```python
from build123d import *

# Parameters (mm, degrees)
SKETCH1_W                      = 11
SKETCH1_H                      = 9
BOSS_EXTRUDE1_DEPTH            = 2.5
BOSS_EXTRUDE2_DEPTH            = 0.4
CUT_EXTRUDE1_DEPTH             = 12.41315031
SKETCH4_W                      = 9
SKETCH4_H                      = 11
BOSS_EXTRUDE3_DEPTH            = 2.45
SKETCH5_W                      = 9
SKETCH5_H                      = 11
BOSS_EXTRUDE4_DEPTH            = 9.45
SKETCH6_W                      = 0.9
SKETCH6_H                      = 8.5
CUT_EXTRUDE2_DEPTH             = 20.892712233
SKETCH7_W                      = 0.52
SKETCH7_H                      = 6
CUT_EXTRUDE3_DEPTH             = 18.424695119
SKETCH8_W                      = 5.62
SKETCH8_H                      = 3
BOSS_EXTRUDE5_DEPTH            = 0.36
SKETCH9_W                      = 3
SKETCH9_H                      = 2.5
BOSS_EXTRUDE6_DEPTH            = 0.52
CUT_EXTRUDE4_REACH             = 19.516
SKETCH11_W                     = 1
SKETCH11_H                     = 0.1
BOSS_EXTRUDE7_DEPTH            = 0.36
CUT_EXTRUDE5_REACH             = 20.109
SKETCH14_W                     = 0.36
SKETCH14_H                     = 1
SKETCH15_W                     = 10
SKETCH15_H                     = 4.5
CUT_EXTRUDE6_DEPTH             = 20.7068516
BOSS_EXTRUDE8_DEPTH            = 10
SKETCH17_W                     = 1.5
SKETCH17_H                     = 1.7
CUT_EXTRUDE7_DEPTH             = 20.7068516
SKETCH18_W                     = 6
SKETCH18_H                     = 1.5
BOSS_EXTRUDE9_DEPTH            = 1.5
BOSS_EXTRUDE10_DEPTH           = 0.25
F_6_5_6_5_DIAMETER_HOLE1_D     = 6.5
F_6_5_6_5_DIAMETER_HOLE1_DEPTH = 7
DRAFT1_ANGLE                   = -47
DRAFT2_ANGLE                   = 47
SKETCH22_W                     = 6
SKETCH22_H                     = 1.25
CHAMFER1_SIZE                  = 0.2


with BuildPart() as part:
    # Sketch1 → Boss-Extrude1 (new body)
    with BuildSketch(Plane(origin=(-11.95, 0, 0), x_dir=(0, -1, 0), z_dir=(-1, 0, 0))):
        with Locations((1, 0)):
            Rectangle(SKETCH1_W, SKETCH1_H)
    extrude(amount=-BOSS_EXTRUDE1_DEPTH)

    # Sketch2 → Boss-Extrude2 (add)
    with BuildSketch(Plane(origin=(0, 0, -4.5), x_dir=(-1, 0, 0), z_dir=(0, 0, -1))):
        with BuildLine():
            Line((10.2, -9.5), (10.2, -7.004276533))
            Line((10.2, -7.004276533), (9.45, -6.2))
            Line((9.45, -6.2), (9.45, 4.5))
            Line((9.45, 4.5), (11.95, 4.5))
            Line((11.95, 4.5), (11.95, -6.2))
            Line((11.95, -6.2), (11.2, -7.004276533))
            Line((11.2, -7.004276533), (11.2, -9.5))
            ThreePointArc((11.2, -9.5), (10.7, -10), (10.2, -9.5))
        make_face()
    extrude(amount=BOSS_EXTRUDE2_DEPTH)

    # Sketch3 → Cut-Extrude1 (cut, through all)
    with BuildSketch(Plane(origin=(-9.45, 0, 0), x_dir=(0, 0, -1), z_dir=(1, 0, 0))):
        with BuildLine():
            Line((4.9, 4.5), (4.5, 4.5))
            Line((4.5, 4.5), (4.5, -3.5))
            ThreePointArc((4.5, -3.5), (4.787298335, -3.673670183), (4.9, -3.989897949))
            Line((4.9, -3.989897949), (4.9, 4.5))
        make_face()
    extrude(amount=-CUT_EXTRUDE1_DEPTH, mode=Mode.SUBTRACT)

    # Sketch4 → Boss-Extrude3 (add)
    with BuildSketch(Plane.ZY.offset(11.95)):
        with Locations((0, -1)):
            Rectangle(SKETCH4_W, SKETCH4_H)
    extrude(amount=BOSS_EXTRUDE3_DEPTH)

    # Sketch5 → Boss-Extrude4 (add)
    with BuildSketch(Plane(origin=(-9.45, 0, 0), x_dir=(0, 0, -1), z_dir=(1, 0, 0))):
        with Locations((0, -1)):
            Rectangle(SKETCH5_W, SKETCH5_H)
    extrude(amount=BOSS_EXTRUDE4_DEPTH)

    # Sketch6 → Cut-Extrude2 (cut, through all)
    with BuildSketch(Plane.XY.offset(4.5)):
        with Locations((-13.95, 0.25)):
            Rectangle(SKETCH6_W, SKETCH6_H)
    extrude(amount=-CUT_EXTRUDE2_DEPTH, mode=Mode.SUBTRACT)

    # Sketch7 → Cut-Extrude3 (cut, through all)
    with BuildSketch(Plane(origin=(0, -4, 0), x_dir=(-1, 0, 0), z_dir=(0, 1, 0))):
        with Locations((14.14, -1.5)):
            Rectangle(SKETCH7_W, SKETCH7_H)
    extrude(amount=-CUT_EXTRUDE3_DEPTH, mode=Mode.SUBTRACT)

    # Sketch8 → Boss-Extrude5 (add)
    with BuildSketch(Plane(origin=(-13.88, 0, 0), x_dir=(0, -1, 0), z_dir=(-1, 0, 0))):
        with Locations((1.19, 0)):
            Rectangle(SKETCH8_W, SKETCH8_H)
    extrude(amount=-BOSS_EXTRUDE5_DEPTH)

    # Sketch9 → Boss-Extrude6 (add)
    with BuildSketch(Plane.ZY.offset(13.88)):
        with Locations((-3, -5.25)):
            Rectangle(SKETCH9_W, SKETCH9_H)
    extrude(amount=BOSS_EXTRUDE6_DEPTH)

    # Sketch11 → Cut-Extrude4 (cut, up to next)
    with BuildSketch(Plane(origin=(-13.52, 0, 0), x_dir=(0, 0, -1), z_dir=(1, 0, 0)), mode=Mode.PRIVATE) as cut_extrude4_sk1:
        with Locations((1, -6.45)):
            Rectangle(SKETCH11_W, SKETCH11_H)
    cut_extrude4_tool1 = extrude(cut_extrude4_sk1.sketch, amount=-CUT_EXTRUDE4_REACH, mode=Mode.PRIVATE) & part.part
    add(cut_extrude4_tool1.solids().sort_by_distance((-13.52, -6.45, -1))[0], mode=Mode.SUBTRACT)

    # Sketch12 → Boss-Extrude7 (add)
    with BuildSketch(Plane(origin=(-13.88, 0, 0), x_dir=(0, -1, 0), z_dir=(-1, 0, 0))):
        with BuildLine():
            Line((9.5, 0.5), (6.5, 0.5))
            Line((6.5, 0.5), (6.5, -0.5))
            Line((6.5, -0.5), (9.5, -0.5))
            ThreePointArc((9.5, -0.5), (10, 0), (9.5, 0.5))
        make_face()
    extrude(amount=-BOSS_EXTRUDE7_DEPTH)

    # Sketch14 → Cut-Extrude5 (cut, up to next)
    with BuildSketch(Plane(origin=(0, -5.32763129, 0), x_dir=(1, 0, 0), z_dir=(0, 1, 0)), mode=Mode.PRIVATE) as cut_extrude5_sk1:
        with Locations((-13.7, -1)):
            Rectangle(SKETCH14_W, SKETCH14_H)
    cut_extrude5_tool1 = extrude(cut_extrude5_sk1.sketch, amount=-CUT_EXTRUDE5_REACH, mode=Mode.PRIVATE) & part.part
    add(cut_extrude5_tool1.solids().sort_by_distance((-13.7, -5.327631, 1))[0], mode=Mode.SUBTRACT)

    # Sketch15 → Cut-Extrude6 (cut, through all)
    with BuildSketch(Plane(origin=(0, 0, -4.5), x_dir=(-1, 0, 0), z_dir=(0, 0, -1))):
        with Locations((8.5, 2.25)):
            Rectangle(SKETCH15_W, SKETCH15_H)
    extrude(amount=-CUT_EXTRUDE6_DEPTH, mode=Mode.SUBTRACT)

    # Sketch16 → Boss-Extrude8 (add)
    with BuildSketch(Plane.ZY.offset(3.5)):
        with BuildLine():
            Line((4.1, 0), (-4.1, 0))
            ThreePointArc((-4.1, 0), (0, 4.1), (4.1, 0))
        make_face()
    extrude(amount=BOSS_EXTRUDE8_DEPTH)

    # Sketch17 → Cut-Extrude7 (cut, through all)
    with BuildSketch(Plane(origin=(0, 0, -4.5), x_dir=(-1, 0, 0), z_dir=(0, 0, -1))):
        with Locations((1.75, 3.65)):
            Rectangle(SKETCH17_W, SKETCH17_H)
    extrude(amount=-CUT_EXTRUDE7_DEPTH, mode=Mode.SUBTRACT)

    # Sketch18 → Boss-Extrude9 (add)
    with BuildSketch(Plane(origin=(-2.5, 0, 0), x_dir=(0, 0, -1), z_dir=(1, 0, 0))):
        with Locations((0, 3.55)):
            Rectangle(SKETCH18_W, SKETCH18_H)
    extrude(amount=BOSS_EXTRUDE9_DEPTH)

    # Sketch19 → Boss-Extrude10 (add)
    with BuildSketch(Plane(origin=(-7.825, 0, 0), x_dir=(0, -1, 0), z_dir=(-1, 0, 0))):
        with BuildLine():
            Line((9.5, 0.5), (6.5, 0.5))
            Line((6.5, 0.5), (6.5, -0.5))
            Line((6.5, -0.5), (9.5, -0.5))
            ThreePointArc((9.5, -0.5), (10, 0), (9.5, 0.5))
        make_face()
    extrude(amount=-BOSS_EXTRUDE10_DEPTH)

    # Ø6.5 (6.5) Diameter Hole1
    with Locations(Plane(origin=(0, 0, 0), x_dir=(0, 0, -1), z_dir=(1, 0, 0))):
        with Locations((0, 0)):
            Hole(F_6_5_6_5_DIAMETER_HOLE1_D / 2, depth=F_6_5_6_5_DIAMETER_HOLE1_DEPTH)

    # Draft1
    draft1_faces = [part.faces().sort_by_distance(p)[0] for p in [
        (-13.7, -5.32763129, 1),
    ]]
    draft(draft1_faces, Plane(origin=(-14.4, -10, 1.5), x_dir=(-1, 0, 0), z_dir=(0, 0, -1)), DRAFT1_ANGLE)

    # Draft2
    draft2_faces = [part.faces().sort_by_distance(p)[0] for p in [
        (-13.7, -6.4, -1),
    ]]
    draft(draft2_faces, Plane(origin=(-14.884987562, -6.4, -0.5), x_dir=(-1, 0, 0), z_dir=(0, 0, -1)), DRAFT2_ANGLE)

    # Sketch22 → Revolve1 (revolve)
    with BuildSketch(Plane.XY, mode=Mode.PRIVATE) as revolve1_sk:
        with Locations((-4, 0.625)):
            Rectangle(SKETCH22_W, SKETCH22_H)
    revolve(revolve1_sk.sketch.rotate(Axis((-7, 0, 0), (1, 0, 0)), 270), axis=Axis((-7, 0, 0), (1, 0, 0)))

    # Chamfer1
    chamfer1_edges = [part.edges().sort_by_distance(p)[0] for p in [
        (-1, 0, 1.25),
    ]]
    chamfer(chamfer1_edges, length=CHAMFER1_SIZE)


solid = part.part
```
The model under review builds one solid part; all positions refer to its coordinate system, in mm. A direction names the side the tool comes from. Give positions to 0.01 mm unless a question says otherwise; leave off trailing zeros. Write each loop counter-clockwise with the first axis right and the second up, starting at its lowest first coordinate (ties: lowest second). Pieces come first, ordered by that corner, then holes.
(1) For P1, Ø1.4, axis at y = 4, z = 0.5, coming from the -X side; P2, Ø1.5, axis at y = 2, z = 1, coming from the +X side; P3, Ø1.7, axis at y = 0, z = -0.5, coming from the +X side, all flat-tipped, find the tip position at first contact; note any pin that passes through.
(2) To check wall thickness, follow L1, parallel to Y at x = -5, z = 0; L2, parallel to X at y = -4.5, z = 0; L3, parallel to Z at x = -4.5, y = -0.25. State the ranges of each line that lie inside material, in increasing order.
(3) Consider section A-A, the plane y = -8.5. Give the boundary of the cut face in (x, z) (3 decimals), and give its area (3 significant figures).
(4) Consider section D-D, the plane y = -2. Give the boundary of the cut face in (x, z).
(5) Consider section B-B, the plane x = -3. Give the boundary of the cut face in (y, z), and give its area (3 significant figures).
(6) The part is to be moulded in two halves that separate along Z. For faces 1 (the flat face through (-13.697, -5.871, -0.993)), 2 (the flat face through (-14, -6, 1.5)), 3 (the flat face through (-2, 2.8, -4)), 4 (the flat face through (-11, -8, -4.5)), say which applies: released by +Z, released by -Z, zero draft, split by the parting line, or undercut.
(7) Tool access review of faces 5 (the cylindrical face through (-8.4, 4.1, -0.1)), 6 (the flat face through (-2, 2.8, 4)), 7 (the flat face through (-13.52, -8, 0)), 8 (the cylindrical face through (-3.549, -1.978, -2.579)), 9 (the flat face through (-2, 4, -3)): name each direction out of +Z, -Z, +X, -X, +Y, -Y from which nothing blocks a thin tool from reaching the whole face with its end or side.
Returned:
1. P1: stops at x = -13.5
1. P2: stops at x = -7
1. P3: stops at x = -1
2. L1: y = -6.5 to -3.25, -1.25 to 1.25, 3.25 to 4.1
2. L2: x = -13.88 to 0
2. L3: z = -4.5 to -3.24, -1.22 to 1.22, 3.24 to 4.5
3. outline: (-13.88, -0.5) - (-13.52, -0.5) - (-13.52, 0.5) - (-13.88, 0.5) - close; (-11.2, -4.9) - (-10.2, -4.9) - (-10.2, -4.5) - (-11.2, -4.5) - close; (-7.825, -0.5) - (-7.575, -0.5) - (-7.575, 0.5) - (-7.825, 0.5) - close
3. area: 1.01 mm2
4. outline: (-13.88, -1.5) - (-13.52, -1.5) - (-13.52, 1.5) - (-13.88, 1.5) - close; (-13.5, -4.5) - (0, -4.5) - (0, -2.56) - (-7, -2.56) - (-7, 2.56) - (0, 2.56) - (0, 4.5) - (-13.5, 4.5) - close
5. outline: (-6.5, -4.5) - (4.5, -4.5) - (4.5, 4.5) - (-6.5, 4.5) - close; circle Ø2.5 at (0, 0); hole circle Ø6.5 at (0, 0)
5. area: 70.7 mm2
6. face 1: undercut
6. face 2: undercut
6. face 3: zero draft
6. face 4: released by +Z
7. face 5: -X, +Y
7. face 6: +Z, +Y
7. face 7: +Z, -Z, -Y
7. face 8: +X
7. face 9: -Z, +Y
